The model under review builds one solid part; all positions refer to its coordinate system, in mm. Coordinates: 2 decimals unless noted, no trailing zeros.
```python
from build123d import *

# Parameters (mm, degrees)
F0_W      = 101.6
F0_H      = 101.6
F1_DEPTH  = 25.4
F1_FACE_W = 101.6
F1_FACE_H = 101.6
F6_D      = 12.7
F6_DEPTH  = 50.8
F6_TIP    = 3.8154649308


with BuildPart() as f1:
    # F0 (on Front) → F1 (new body)
    with BuildSketch(Plane.XZ):
        with Locations((50.8, 50.8)):
            Rectangle(F0_W, F0_H)
    extrude(amount=F1_DEPTH)

    # F3 (on offset) → F4 section 0
    with BuildSketch(Plane.XZ.offset(374.65)):
        Polygon((50.8, 101.6), (0, 50.8), (50.8, 0), (101.6, 50.8), align=None)
    # F1_face (on face) → F4 section 1
    with BuildSketch(Plane(origin=(50.8, -25.4, 50.8), x_dir=(1, 0, 0), z_dir=(0, -1, 0))):
        Rectangle(F1_FACE_W, F1_FACE_H)
    loft()

    # F6
    with Locations(Plane.XZ.offset(374.65)):
        with Locations((50.8, 50.8)):
            Hole(F6_D / 2, depth=F6_DEPTH)
            with Locations((0, 0, -(F6_DEPTH + F6_TIP / 2))):  # 118° drill point
                Cone(0, F6_D / 2, F6_TIP, mode=Mode.SUBTRACT)


solid = f1.part
```
(1) Wall thickness on probe 1 along X at (y, z) = (-339, 50.8); probe 2 along X at (y, z) = (-336, 50.8); probe 3 along Z at (x, y) = (50, -358): over which ranges is each line inside the solid? List them lowest first.
A:
probe 1: x = 4.22 to 44.45, 57.15 to 97.38
probe 2: x = 4.5 to 44.45, 57.15 to 97.1
probe 3: z = 2.93 to 44.5, 57.1 to 100.13
(2) Draft analysis for pull direction X (two halves, no side actions). For faces 1 (the face through (61, -374.65, 52)), 2 (the face through (101.6, -13, 50)), 3 (the face through (0, -13, 50)), 4 (the face through (44.743, -348.894, 52.707)), state which applies: released by +X, released by -X, zero draft, split by the parting line, or undercut.
A:
face 1: zero draft
face 2: released by +X
face 3: released by -X
face 4: undercut
(3) For pin 1 Ø5 at (x, y) = (89.5, -264.5) entering from -Z; pin 2 Ø10 at (x, y) = (49.5, -318.5) entering from -Z; pin 3 Ø6 at (x, y) = (87, -259.5) entering from +Z, all flat-tipped, find the tip position at first contact; note any pin that passes through.
A:
pin 1: stops at z = 38.77
pin 2: stops at z = 3.2
pin 3: stops at z = 76.44
